```python
from build123d import *

# Parameters (mm, degrees)
F0_W     = 38.1
F0_H     = 31.75
F1_DEPTH = 25.4
F2_W     = 5.603711
F2_H     = 6.35
F3_DEPTH = 25.4


with BuildPart() as f1:
    # F0 (on Front) → F1 (new body)
    with BuildSketch(Plane.XZ):
        with Locations((19.05, 15.875)):
            Rectangle(F0_W, F0_H)
    extrude(amount=F1_DEPTH)

    # F2 (on face) → F3 (cut)
    with BuildSketch(Plane.XZ.offset(25.4)):
        with Locations((19.020174, 3.175)):
            Rectangle(F2_W, F2_H)
        Polygon((0, 31.75), (0, 0), (12.7, 31.75), align=None)
        Polygon((25.229283, 31.75), (38.1, 0), (38.1, 31.75), align=None)
    extrude(amount=-F3_DEPTH, mode=Mode.SUBTRACT)


solid = f1.part
```
Verification items for the finished model (mm, model axes). A direction names the side the tool comes from. Coordinates: 2 decimals unless noted, no trailing zeros. Write each loop counter-clockwise with the first axis right and the second up, starting at its lowest first coordinate (ties: lowest second). Pieces come first, ordered by that corner, then holes. Notation, with made-up numbers: (48.5, 83.25) - (78.5, 83.25) arc R31 ccw to (78.5, 118.25) - close; hole circle Ø10 at (4.5, -31). An arc over 180 degrees is marked (long way). Write item = value, one per line.
Q1. Cross-section at A-A (z = 3). Enter the section's corners in (x, y), plus the area to 3 significant figures.
Answer:
outline = (1.2, -25.4) - (16.22, -25.4) - (16.22, 0) - (1.2, 0) - close; (21.82, -25.4) - (36.88, -25.4) - (36.88, 0) - (21.82, 0) - close
area = 764 mm²
Q2. Cross-section at B-B (y = -1.5). Enter the section's corners in (x, z).
Answer:
outline = (0, 0) - (16.22, 0) - (16.22, 6.35) - (21.82, 6.35) - (21.82, 0) - (38.1, 0) - (25.23, 31.75) - (12.7, 31.75) - close
Q3. Material ranges on L1, parallel to X at y = -7.25, z = 3.5; L2, parallel to Z at x = 17, y = -6.5; L3, parallel to X at y = -24.5, z = 30, recorded low to high. Write a range as from..to.
Answer:
L1 = 1.4..16.22, 21.82..36.68
L2 = 6.35..31.75
L3 = 12..25.94
Q4. Mould release check, pull along X, two halves, no side actions. Record for faces 1 (the face through (31.575, -12.878, 16.097)), 2 (the face through (19, -13, 31.75)), 3 (the face through (19, -13, 6.35)), 4 (the face through (6.26, -12.88, 15.65)): released by +X, released by -X, zero draft, split by the parting line, or undercut.
Answer:
face_1 = released by +X
face_2 = zero draft
face_3 = undercut
face_4 = released by -X
Q5. Access from +Z, -Z, +X, -X, +Y, -Y to the whole of each face (thin tool, end or side, straight path). Record for faces 5 (the face through (19, 0, 13)), 6 (the face through (21.822, -13, 3)).
Answer:
face_5 = +Z, -Z, +X, -X, +Y
face_6 = -Z, +Y, -Y
Q6. Cross-section at C-C (x = 19). Enter the section's corners in (y, z), plus the area to 3 significant figures.
Answer:
outline = (-25.4, 6.35) - (0, 6.35) - (0, 31.75) - (-25.4, 31.75) - close
area = 645 mm²
Q7. Go/stop test with flat-tipped pins: pin 1 Ø1.5 at (x, y) = (27.5, -12.5) entering from -Z; pin 2 Ø3 at (y, z) = (-13.5, 3) entering from -X; pin 3 Ø1 at (x, y) = (12, -11.5) entering from +Z; pin 4 Ø3 at (y, z) = (-11, 4.5) entering from +X. Record where each tip stops, or that it passes through.
Answer:
pin_1 = 0
pin_2 = 0.6
pin_3 = 31.25
pin_4 = 36.88
Q8. Cross-section at D-D (z = 20.5). Enter the section's corners in (x, y), plus the area to 3 significant figures.
Answer:
outline = (8.2, -25.4) - (29.79, -25.4) - (29.79, 0) - (8.2, 0) - close
area = 548 mm²
